```python
from build123d import *

# Parameters (mm, degrees)
SKETCH_1_W                = 35
SKETCH_1_H                = 15
EXTRUDE_1_DEPTH           = 4
HOLE_WIZARD_3_5_3_5_1_D   = 3.5
HOLE_WIZARD_1_D           = 4.5
HOLE_WIZARD_1_CBORE_D     = 8
HOLE_WIZARD_1_CBORE_DEPTH = 1
CUT_EXTRUDE_1_DEPTH       = 2


with BuildPart() as part:
    # 草圖1 → 填料-伸長1 (new body)
    with BuildSketch(Plane(origin=(0, 0, 0), x_dir=(1, 0, 0), z_dir=(0, 1, 0))):
        with Locations((17.5, 7.5)):
            Rectangle(SKETCH_1_W, SKETCH_1_H)
    extrude(amount=EXTRUDE_1_DEPTH)

    # Ø3.5 (3.5) 直徑孔1 (through all)
    with Locations(Plane(origin=(0, 4, 0), x_dir=(1, 0, 0), z_dir=(0, 1, 0))):
        with Locations((17.5, 7.5)):
            Hole(HOLE_WIZARD_3_5_3_5_1_D / 2)

    # 鑽孔1 (through all)
    with Locations(Plane(origin=(0, 4, 0), x_dir=(1, 0, 0), z_dir=(0, 1, 0))):
        with Locations((6, 7.5), (29, 7.5)):
            CounterBoreHole(HOLE_WIZARD_1_D / 2, HOLE_WIZARD_1_CBORE_D / 2, HOLE_WIZARD_1_CBORE_DEPTH)

    # 草圖8 → 除料-伸長1 (cut)
    with BuildSketch(Plane.XZ):
        Polygon((17.5, -10.675426481), (20.25, -9.08771324), (20.25, -5.91228676), (17.5, -4.324573519), (14.75, -5.91228676), (14.75, -9.08771324), align=None)
    extrude(amount=-CUT_EXTRUDE_1_DEPTH, mode=Mode.SUBTRACT)


solid = part.part
```
Design review of the part built by this model. Coordinates are the model's own, in mm. A direction names the side the tool comes from. Give positions to 0.01 mm unless a question says otherwise; leave off trailing zeros. Order: outer loops, then holes, each group sorted by start corner. A loop starts at its lowest first (then second) coordinate and runs counter-clockwise, first axis right, second up. Notation, with made-up numbers: (74.5, -7) - (116.5, -7) arc R17 ccw to (116.5, -1) - close; hole circle Ø11 at (-9, 71). An arc over 180 degrees is marked (long way). Use a Markdown table: item, result. Add a question column.
(1) Add section C-C on y = 1.45. Give the boundary of the cut face in (x, z), then the cut area to 3 significant figures.
(2) Add section A-A on z = -7.5. Give the boundary of the cut face in (x, y), then the cut area to 3 significant figures.
(3) Wall thickness on probe 1 along Z at (x, y) = (6, 3.65); probe 2 along X at (y, z) = (2.1, -6.5); probe 3 along X at (y, z) = (2.5, -8): over which ranges is each line inside the solid? List them lowest first. Write a range as [from, to].
(4) Add section B-B on x = 29. Give the boundary of the cut face in (y, z).
(5) Mouldability with a two-part tool opening along Z and no side actions: class faces 1 (the face through (16.106, 0.986, -9.87)), 2 (the face through (17, 2, 0)), 3 (the face through (17, 2, -15)) as +Z half, -Z half, draft (parallel to the pull), parting line (faces both ways), or undercut.
(6) Clearance check with a flat-ended pin moving along its axis: P1, Ø4, axis at x = 30.5, z = -7.5, coming from the +Y side. State where the tip first meets the part, or that it passes through.
(7) Machinability: for faces 4 (the face through (0, 2, -7)), 5 (the face through (8, 3, -6)), 6 (the face through (16.14, 0.99, -5.11)), which of the approach directions +Z, -Z, +X, -X, +Y, -Y give a long, thin tool a straight path to every point of the face, cutting with its end or side? Answer none if there is none.
Report:
| question | item | result |
|---|---|---|
| 1 | outline | (0, -15) - (35, -15) - (35, 0) - (0, 0) - close; hole circle Ø4.5 at (6, -7.5); hole (14.75, -9.09) - (17.5, -10.68) - (20.25, -9.09) - (20.25, -5.91) - (17.5, -4.32) - (14.75, -5.91) - close; hole circle Ø4.5 at (29, -7.5) |
| 1 | area | 467 mm² |
| 2 | outline | (0, 0) - (3.75, 0) - (3.75, 3) - (2, 3) - (2, 4) - (0, 4) - close; (8.25, 0) - (14.75, 0) - (14.75, 2) - (15.75, 2) - (15.75, 4) - (10, 4) - (10, 3) - (8.25, 3) - close; (19.25, 2) - (20.25, 2) - (20.25, 0) - (26.75, 0) - (26.75, 3) - (25, 3) - (25, 4) - (19.25, 4) - close; (31.25, 0) - (35, 0) - (35, 4) - (33, 4) - (33, 3) - (31.25, 3) - close |
| 2 | area | 79.0 mm² |
| 3 | probe 1 | z = [-15, -11.5], [-3.5, 0] |
| 3 | probe 2 | x = [0, 3.98], [8.02, 16.06], [18.94, 26.98], [31.02, 35] |
| 3 | probe 3 | x = [0, 3.81], [8.19, 15.82], [19.18, 26.81], [31.19, 35] |
| 4 | outline | (0, -15) - (4, -15) - (4, -11.5) - (3, -11.5) - (3, -9.75) - (0, -9.75) - close; (0, -5.25) - (3, -5.25) - (3, -3.5) - (4, -3.5) - (4, 0) - (0, 0) - close |
| 5 | face 1 | undercut |
| 5 | face 2 | +Z half |
| 5 | face 3 | -Z half |
| 6 | P1 | stops at y = 3 |
| 7 | face 4 | +Z, -Z, -X, +Y, -Y |
| 7 | face 5 | +Y |
| 7 | face 6 | -Y |
